```python
from build123d import *

# Parameters (mm, degrees)
F0_R     = 3
F1_DEPTH = 2
F2_W     = 4
F2_H     = 25
F3_DEPTH = 70
F4_R     = 2.75
F5_DEPTH = 40.501
F6_R     = 12.49999


# Not quite as in the source:
# - a fillet or chamfer is up to 0.001 mm smaller than in the source, because OpenCascade refuses the exact size


with BuildPart() as f1:
    # F0 (on Top) → F1 (new body)
    with BuildSketch(Plane.XY):
        with BuildLine():
            ThreePointArc((0, -12.5), (8.8388347648, -8.8388347648), (12.5, 0))
            ThreePointArc((12.5, 0), (8.8388347648, 8.8388347648), (0, 12.5))
            ThreePointArc((0, 12.5), (-12.5, 0), (0, -12.5))
        make_face()
        with BuildLine():
            ThreePointArc((0, 9.5), (6.1662175321, 7.2268777039), (9.3815789474, 1.4953181783))
            ThreePointArc((9.3815789474, 1.4953181783), (10.5179313388, 1.1017330845), (11, 0))
            ThreePointArc((11, 0), (10.5179313388, -1.1017330845), (9.3815789474, -1.4953181783))
            ThreePointArc((9.3815789474, -1.4953181783), (6.1662175364, -7.2268777002), (1.13e-08, -9.5))
            ThreePointArc((1.13e-08, -9.5), (-6.1662175278, -7.2268777076), (-9.3815789474, -1.4953181783))
            ThreePointArc((-9.3815789474, -1.4953181783), (-11, 0), (-9.3815789474, 1.4953181783))
            ThreePointArc((-9.3815789474, 1.4953181783), (-6.1662175321, 7.2268777039), (0, 9.5))
        make_face(mode=Mode.SUBTRACT)
        with BuildLine():
            ThreePointArc((1.4933936552, -7.859375), (6.1622702489, -5.1016100771), (8, 0))
            ThreePointArc((8, 0), (6.1622702489, 5.1016100771), (1.4933936552, 7.859375))
            ThreePointArc((1.4933936552, 7.859375), (0, 6.5), (-1.4933936552, 7.859375))
            ThreePointArc((-1.4933936552, 7.859375), (-6.1622702489, 5.1016100771), (-8, 0))
            ThreePointArc((-8, 0), (-6.1622702489, -5.1016100771), (-1.4933936552, -7.859375))
            ThreePointArc((-1.4933936552, -7.859375), (0, -6.5), (1.4933936552, -7.859375))
        make_face()
        Circle(F0_R, mode=Mode.SUBTRACT)
        with BuildLine():
            ThreePointArc((0, 12.5), (8.8388347648, 8.8388347648), (12.5, 0))
            ThreePointArc((12.5, 0), (8.8388347648, -8.8388347648), (0, -12.5))
            Line((0, -12.5), (28, -12.5))
            Line((28, -12.5), (28, 12.5))
            Line((28, 12.5), (0, 12.5))
        make_face()
        with BuildLine():
            ThreePointArc((-1.4933936552, 7.859375), (-1.1092649593, 9.0097184013), (0, 9.5))
            ThreePointArc((0, 9.5), (-6.1662175321, 7.2268777039), (-9.3815789474, 1.4953181783))
            ThreePointArc((-9.3815789474, 1.4953181783), (-8.3982669155, 1.0179313388), (-8, 0))
            ThreePointArc((-8, 0), (-6.1622702489, 5.1016100771), (-1.4933936552, 7.859375))
        make_face()
        with BuildLine():
            ThreePointArc((8, 0), (8.3982669155, 1.0179313388), (9.3815789474, 1.4953181783))
            ThreePointArc((9.3815789474, 1.4953181783), (6.1662175321, 7.2268777039), (0, 9.5))
            ThreePointArc((0, 9.5), (1.0606601718, 9.0606601718), (1.5, 8))
            ThreePointArc((1.5, 8), (1.4983475036, 7.9296099538), (1.4933936552, 7.859375))
            ThreePointArc((1.4933936552, 7.859375), (6.1622702489, 5.1016100771), (8, 0))
        make_face()
        with BuildLine():
            ThreePointArc((1.13e-08, -9.5), (6.1662175364, -7.2268777002), (9.3815789474, -1.4953181783))
            ThreePointArc((9.3815789474, -1.4953181783), (8.3982669155, -1.0179313388), (8, 0))
            ThreePointArc((8, 0), (6.1622702489, -5.1016100771), (1.4933936552, -7.859375))
            ThreePointArc((1.4933936552, -7.859375), (1.4983475036, -7.9296099538), (1.5, -8))
            ThreePointArc((1.5, -8), (1.0606601758, -9.0606601678), (1.13e-08, -9.5))
        make_face()
        with BuildLine():
            ThreePointArc((-9.3815789474, -1.4953181783), (-6.1662175278, -7.2268777076), (1.13e-08, -9.5))
            ThreePointArc((1.13e-08, -9.5), (-1.1092649555, -9.0097184055), (-1.4933936552, -7.859375))
            ThreePointArc((-1.4933936552, -7.859375), (-6.1622702489, -5.1016100771), (-8, 0))
            ThreePointArc((-8, 0), (-8.3982669155, -1.0179313388), (-9.3815789474, -1.4953181783))
        make_face()
    extrude(amount=F1_DEPTH)

    # F2 (on face) → F3 (join)
    with BuildSketch(Plane.XY.offset(2)):
        with Locations((26, 0)):
            Rectangle(F2_W, F2_H)
    extrude(amount=F3_DEPTH)

    # F4 (on face) → F5 (cut, through all)
    with BuildSketch(Plane.YZ.offset(28)):
        with Locations((0, 59.5)):
            Circle(F4_R)
    extrude(amount=-F5_DEPTH, mode=Mode.SUBTRACT)

    # F6 (radius 12.5 in the source; OpenCascade refuses exactly that, so slightly less here)
    f6_edges = [f1.edges().sort_by_distance(p)[0] for p in [
        (24, 0, 2),
        (26, -12.5, 72),
        (26, 12.5, 72),
    ]]
    fillet(f6_edges, radius=F6_R)


solid = f1.part
```
The listing builds one solid part. Answer for the finished solid, in the listing's coordinates (mm). A direction names the side the tool comes from. Round coordinates to 2 decimals unless told otherwise and drop trailing zeros. Write each loop counter-clockwise with the first axis right and the second up, starting at its lowest first coordinate (ties: lowest second). Pieces come first, ordered by that corner, then holes. Notation, with made-up numbers: (-8, 71) -> (47, 71) arc R15 cw to (47, 89) -> close; hole circle Ø11 at (51.25, 71.5). An arc over 180 degrees is marked (long way). Use CSV: the item, a comma, the result in double quotes. Start each with the question number.
(1) Section C-C on x = 7 is taken. Give the vertices of the cut face in (y, z), then the cut area to 3 significant figures.
(2) Section B-B on y = 4.25 is taken. Give the vertices of the cut face in (x, z).
(3) Section D-D on y = 10.25 is taken. Give the vertices of the cut face in (x, z), then the cut area to 3 significant figures.
(4) Consider L1, parallel to Z at x = 24.85, y = 0; L2, parallel to X at y = -11, z = 34; L3, parallel to Z at x = 4, y = 8.5. Determine where each line is inside the solid, lowest interval first. Write a range as from..to.
(5) The mould has two halves that part along X. Classify faces 1 (the face through (28, 0, 35)), 2 (the face through (24, 0, 43)), 3 (the face through (-3, 0, 1)), 4 (the face through (26.028, -0.358, 62.227)): released by +X, released by -X, zero draft, split by the parting line, or undercut.
(6) Section A-A on z = 42.5 is taken. Give the vertices of the cut face in (x, y).
(7) Each of these flat-tipped pins is pushed along its axis until it touches: pin 1 (12 mm diameter, centred on y = 9.5, z = 50.5, fed in from -X); pin 2 (1.5 mm diameter, centred on x = 7.5, y = 5, fed in from +Z). Where does it stop, or does it pass through?
(8) Which of the six approach directions +Z, -Z, +X, -X, +Y, -Y give full straight-line access (tool end or side, diameter ignored) to faces 5 (the face through (2, -3, 2)), 6 (the face through (24.3, 12.5, 23))?
A:
1,outline,"(-12.5, 0) -> (12.5, 0) -> (12.5, 2) -> (-12.5, 2) -> close"
1,area,"50.0 mm²"
2,outline,"(-11.76, 0) -> (28, 0) -> (28, 71.26) -> (24, 71.26) -> (24, 14.5) arc R12.5 cw to (11.5, 2) -> (-11.76, 2) -> close"
3,outline,"(-7.15, 0) -> (28, 0) -> (28, 66.65) -> (24, 66.65) -> (24, 14.5) arc R12.5 cw to (11.5, 2) -> (-7.15, 2) -> close"
3,area,"362 mm²"
4,L1,"z = 0..56.75, 62.25..72"
4,L2,"x = 24..28"
4,L3,"z = 0..2"
5,face 1,"released by +X"
5,face 2,"released by -X"
5,face 3,"undercut"
5,face 4,"zero draft"
6,outline,"(24, -12.5) -> (28, -12.5) -> (28, 12.5) -> (24, 12.5) -> close"
7,pin 1,"stops at x = 24"
7,pin 2,"stops at z = 2"
8,face 5,"+Z, -X, +Y, -Y"
8,face 6,"+Z, -Z, +X, -X, +Y"
